Input: part model. Units: mm. Frame: model coordinates. A direction names the side the tool comes from. Round coordinates to 2 decimals unless told otherwise and drop trailing zeros. Loops run counter-clockwise (first coordinate to the right, second up) from the corner with the lowest first, then second, coordinate; pieces in that order, holes last. Notation, with made-up numbers: (13.25, -28) -> (25.25, -28) arc R25 ccw to (25.25, -14) -> close; hole circle Ø8 at (33, 66). An arc over 180 degrees is marked (long way). One line per question, with ' | ' between items. Start each with the question number.
Q1. Material intervals for L1, parallel to Y at x = 0, z = 19; L2, parallel to Z at x = 7.25, y = 1.25, sorted ascending.
Q2. Cut plane C-C on z = 8. Return loops of the section in (x, y), and give its area (3 significant figures).
Q3. Access query for faces 5 (the face through (-2, -8, 4)), 6 (the face through (10, 3.2, 2)). Directions: +Z, -Z, +X, -X, +Y, -Y. A direction counts if a zero-diameter tool reaches every point of the face in a straight line with its end or side. Return the directions, or none.
Q4. Cut plane D-D on y = -3.25. Return loops of the section in (x, z), and give its area (3 significant figures).
Q5. Cut plane A-A on x = 0. Return loops of the section in (y, z), and give its area (3 significant figures).
Q6. Mould query, pull axis Y, two halves, no side actions, for faces 1 (the face through (0, 0, 44)), 2 (the face through (-1.5, -0.07, 19.23)), 3 (the face through (-1.73, -7.81, 21.26)), 4 (the face through (0, 0, 39)). Classes: pulls with the +Y half, pulls with the -Y half, needs draft (parallel to the pull), parting line crosses it, or undercut.
Q7. Contact query for flat-ended pins moving along their axis: P1, Ø12, axis at y = 5, z = 34.5, coming from the -X side; P2, Ø0.9, axis at x = -0.5, y = -0.5, coming from the -Z side; P3, Ø1, axis at x = 5.5, y = -7.5, coming from the +Z side. Output: stop coordinate, or through.
from build123d import *

# Parameters (mm, degrees)
F0_R     = 10.5
F1_DEPTH = 4
F2_R     = 8
F3_DEPTH = 39
F4_W     = 7
F4_H     = 5
F6_R     = 1.5
F7_DEPTH = 39


with BuildPart() as f1:
    # F0 (on Top) → F1 (new body)
    with BuildSketch(Plane.XY):
        Circle(F0_R)
    extrude(amount=F1_DEPTH)

    # F2 (on Top) → F3 (join)
    with BuildSketch(Plane.XY):
        Circle(F2_R)
    extrude(amount=F3_DEPTH)

    # F4 (on Right) → F5 (revolve)
    with BuildSketch(Plane.YZ):
        with Locations((3.5, 41.5)):
            Rectangle(F4_W, F4_H)
    revolve(axis=Axis((0, 0, 41.5), (0, 0, -1)))

    # F6 (on face) → F7 (cut)
    with BuildSketch(Plane(origin=(0, 0, 0), x_dir=(1, 0, 0), z_dir=(0, 0, -1))):
        Circle(F6_R)
    extrude(amount=-F7_DEPTH, mode=Mode.SUBTRACT)


solid = f1.part
Results:
1) L1: -8 to -1.5, 1.5 to 8 | L2: 0 to 39
2) outline: circle Ø16 at (0, 0); hole circle Ø3 at (0, 0) | area: 194 mm^2
3) face 5: +Z | face 6: +Z, -Z
4) outline: (-9.98, 0) -> (9.98, 0) -> (9.98, 4) -> (7.31, 4) -> (7.31, 39) -> (6.2, 39) -> (6.2, 44) -> (-6.2, 44) -> (-6.2, 39) -> (-7.31, 39) -> (-7.31, 4) -> (-9.98, 4) -> close | area: 654 mm^2
5) outline: (-10.5, 0) -> (-1.5, 0) -> (-1.5, 39) -> (1.5, 39) -> (1.5, 0) -> (10.5, 0) -> (10.5, 4) -> (8, 4) -> (8, 39) -> (7, 39) -> (7, 44) -> (-7, 44) -> (-7, 39) -> (-8, 39) -> (-8, 4) -> (-10.5, 4) -> close | area: 597 mm^2
6) face 1: needs draft | face 2: undercut | face 3: parting line crosses it | face 4: undercut
7) P1: x = -8 | P2: z = 39 | P3: z = 4
